Source: CAD feature listing. Evaluate the final solid. Frame: model axes, mm. Face numbers are marked on the shaded views. Round coordinates to 2 decimals unless told otherwise and drop trailing zeros. Order: outer loops, then holes, each group sorted by start corner. A loop starts at its lowest first (then second) coordinate and runs counter-clockwise, first axis right, second up. Notation, with made-up numbers: M 8,21.5 L 30,21.5 A33 cw 30,54.5 Z; hole C -11,-16 d2. An arc over 180 degrees is marked long. Use one line per item in the form item = value. Start each with the question number.
Q1. Material intervals for probe 1 along Y at (x, z) = (4, 11); probe 2 along X at (y, z) = (-1.5, 46); probe 3 along Z at (x, y) = (-4.5, 11), sorted ascending.
Q2. Contact query for flat-ended pins moving along their axis: pin 1 (1.5 mm diameter, centred on x = 16.5, z = 53.5, fed in from +Y); pin 2 (3 mm diameter, centred on y = -15.5, z = 18.5, fed in from +X); pin 3 (1.5 mm diameter, centred on x = -3.5, z = 52.5, fed in from +Y); pin 4 (10 mm diameter, centred on x = 5, y = -9.5, fed in from +Z). Output: stop coordinate, or through.
Q3. Section C-C (y = 8.5). Return the cut outline in (x, z).
Q4. Pull-direction query (Y, two-part tool) for the marked faces 1, 2 and 3; classes: pulls with the +Y half, pulls with the -Y half, needs draft (parallel to the pull), parting line crosses it, or undercut.
Q5. Section B-B (x = 5). Return the cut outline in (y, z), plus the area to 3 significant figures.
Q6. Section A-A (z = 45). Return the cut outline in (x, y), plus the area to 3 significant figures.
Q7. Section D-D (z = 10.5). Return the cut outline in (x, y).
from build123d import *

# Parameters (mm, degrees)
EXTRUDE_1_DEPTH     = 60
SKETCH_2_R          = 13
CUT_EXTRUDE_1_DEPTH = 18
SKETCH_3_R          = 11.1
CUT_EXTRUDE_2_DEPTH = 53.570516706


with BuildPart() as part:
    # 草图1 → 凸台-拉伸1 (new body)
    with BuildSketch(Plane.XY):
        Polygon((-12.695703738, 19.978799762), (-23.65, -1.005402075), (-10.954296262, -20.984201837), (12.695703738, -19.978799762), (23.65, 1.005402075), (10.954296262, 20.984201837), align=None)
    extrude(amount=EXTRUDE_1_DEPTH)

    # 草图2 → 切除-拉伸1 (cut)
    with BuildSketch(Plane.XY.offset(60)):
        Circle(SKETCH_2_R)
    extrude(amount=-CUT_EXTRUDE_1_DEPTH, mode=Mode.SUBTRACT)

    # 草图3 → 切除-拉伸2 (cut, through all)
    with BuildSketch(Plane.XY.offset(42)):
        Circle(SKETCH_3_R)
    extrude(amount=-CUT_EXTRUDE_2_DEPTH, mode=Mode.SUBTRACT)


solid = part.part
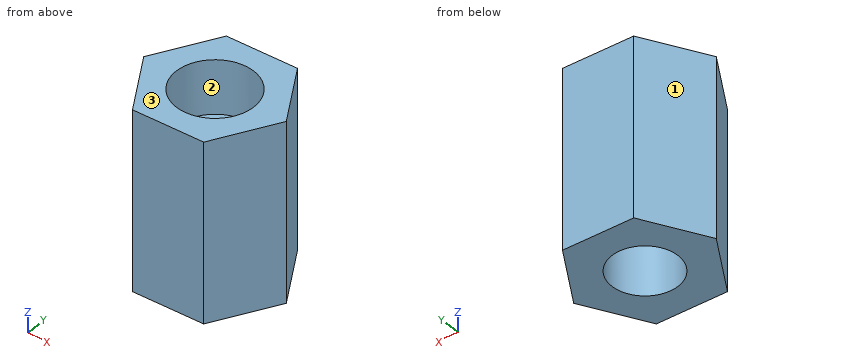
Results list:
q1.probe_1 = -20.35 to -10.35, 10.35 to 20.69
q1.probe_2 = -23.34 to -12.91, 12.91 to 22.34
q1.probe_3 = 0 to 42
q2.pin_1 = 13.44
q2.pin_2 = 15.82
q2.pin_3 = 20.4
q2.pin_4 = 60
q3.outline = M -18.69,0 L -7.14,0 L -7.14,42 L -9.84,42 L -9.84,60 L -18.69,60 Z; M 7.14,0 L 18.89,0 L 18.89,60 L 9.84,60 L 9.84,42 L 7.14,42 Z
q4.face_1 = pulls with the +Y half
q4.face_2 = undercut
q4.face_3 = needs draft
q5.outline = M -20.31,0 L -9.91,0 L -9.91,42 L -12,42 L -12,60 L -20.31,60 Z; M 9.91,0 L 20.73,0 L 20.73,60 L 12,60 L 12,42 L 9.91,42 Z
q5.area = 1,200 mm2
q6.outline = M -23.65,-1.01 L -10.95,-20.98 L 12.7,-19.98 L 23.65,1.01 L 10.95,20.98 L -12.7,19.98 Z; hole C 0,0 d26
q6.area = 925 mm2
q7.outline = M -23.65,-1.01 L -10.95,-20.98 L 12.7,-19.98 L 23.65,1.01 L 10.95,20.98 L -12.7,19.98 Z; hole C 0,0 d22.2
